```python
from build123d import *

# Parameters (mm, degrees)
RESSALTO_EXTRUS_O1_DEPTH = 30
ESBO_O2_W                = 25
ESBO_O2_H                = 20
CORTE_EXTRUS_O1_DEPTH    = 25
ESBO_O3_W                = 20
ESBO_O3_H                = 20
CORTE_EXTRUS_O2_DEPTH    = 10
ESBO_O4_W                = 15
ESBO_O4_H                = 20
CORTE_EXTRUS_O3_DEPTH    = 10


with BuildPart() as part:
    # Esboço1 → Ressalto-extrusão1 (new body)
    with BuildSketch(Plane.XY):
        Polygon((0, 0), (0, 40), (40, 40), (40, 25), (60, 25), (60, 0), align=None)
    extrude(amount=RESSALTO_EXTRUS_O1_DEPTH)

    # Esboço2 → Corte-extrusão1 (cut)
    with BuildSketch(Plane(origin=(0, 40, 0), x_dir=(1, 0, 0), z_dir=(0, 1, 0))):
        with Locations((27.5, -20)):
            Rectangle(ESBO_O2_W, ESBO_O2_H)
    extrude(amount=-CORTE_EXTRUS_O1_DEPTH, mode=Mode.SUBTRACT)

    # Esboço3 → Corte-extrusão2 (cut)
    with BuildSketch(Plane(origin=(0, 25, 0), x_dir=(1, 0, 0), z_dir=(0, 1, 0))):
        with Locations((50, -20)):
            Rectangle(ESBO_O3_W, ESBO_O3_H)
    extrude(amount=-CORTE_EXTRUS_O2_DEPTH, mode=Mode.SUBTRACT)

    # Esboço4 → Corte-extrusão3 (cut)
    with BuildSketch(Plane(origin=(0, 40, 0), x_dir=(1, 0, 0), z_dir=(0, 1, 0))):
        with Locations((7.5, -20)):
            Rectangle(ESBO_O4_W, ESBO_O4_H)
    extrude(amount=-CORTE_EXTRUS_O3_DEPTH, mode=Mode.SUBTRACT)


solid = part.part
```
Part model, mm, in its own coordinate system. A direction names the side the tool comes from. Round coordinates to 2 decimals unless told otherwise and drop trailing zeros. Write each loop counter-clockwise with the first axis right and the second up, starting at its lowest first coordinate (ties: lowest second). Pieces come first, ordered by that corner, then holes.
Item 1: Which spindle directions (+Z, -Z, +X, -X, +Y, -Y) get a long thin tool onto all of the face, cutting with end or side? Do faces 1 (the flat face through (50, 25, 5)), 2 (the flat face through (37, 15, 20)), 3 (the flat face through (7, 30, 20)), 4 (the flat face through (20, 40, 5)). Say none if no direction does.
Results:
face 1: +Z, -Z, +X, +Y
face 2: +Z, +X, +Y
face 3: +Z, +X, -X, +Y
face 4: +Z, -Z, +X, -X, +Y
Item 2: Drop flat-ended pins along their axis: pin 1 Ø3 at (x, y) = (42, 19.5) entering from +Z; pin 2 Ø2 at (x, z) = (48, 26.5) entering from +Y; pin 3 Ø5 at (x, z) = (46.5, 6.5) entering from +Y. Give the stop position or say it passes through.
Results:
pin 1: stops at z = 10
pin 2: stops at y = 15
pin 3: stops at y = 25
Item 3: Cut at A-A, the plane y = 23.5. Give the cut face in (x, z), plus the area to 3 significant figures.
Results:
outline: (0, 0) - (60, 0) - (60, 10) - (15, 10) - (15, 30) - (0, 30) - close
area: 900 mm2
Item 4: Probe L1, parallel to Y at x = 7, z = 21; L2, parallel to Y at x = 32, z = 13; L3, parallel to X at y = 36, z = 3.5. List the from-to ranges inside material, lowest first.
Results:
L1: y = 0 to 30
L2: y = 0 to 15
L3: x = 0 to 40
Item 5: Cut at B-B, the plane x = 23.5. Give the cut face in (y, z), plus the area to 3 significant figures.
Results:
outline: (0, 0) - (40, 0) - (40, 10) - (15, 10) - (15, 30) - (0, 30) - close
area: 700 mm2
